Model file for the job. Use its own axes, mm. A direction names the side the tool comes from. Coordinates: 2 decimals unless noted, no trailing zeros. Loops run counter-clockwise (first coordinate to the right, second up) from the corner with the lowest first, then second, coordinate; pieces in that order, holes last. Notation, with made-up numbers: M 83.25,-38 L 110.25,-38 A24 ccw 110.25,-27 Z; hole C 22.25,2.25 d7. An arc over 180 degrees is marked long. One line per question, with ' | ' between items. Start each with the question number.
```python
from build123d import *

# Parameters (mm, degrees)
SKETCH_1_R      = 5
EXTRUDE_1_DEPTH = 3


with BuildPart() as part:
    # 草图1 → 凸台-拉伸1 (new body)
    with BuildSketch(Plane.XY):
        Polygon((-9.837963803, 8.570517693), (60.162036197, 8.570517693), (-9.837963803, -31.429482307), align=None)
        Circle(SKETCH_1_R, mode=Mode.SUBTRACT)
        Polygon((5.831882272, 4.782203257), (5.831882272, -17.086702804), (46.814556623, 4.782203257), align=None, mode=Mode.SUBTRACT)
    extrude(amount=EXTRUDE_1_DEPTH)


solid = part.part
```
(1) Band-saw the part on D-D on y = -11. Write the cut outline in (x, z).
(2) Band-saw the part on C-C on x = 0. Write the cut outline in (y, z), then the cut area to 3 significant figures.
(3) Drill centre lines: line 1 (X direction, y = -2, z = 1.5); line 2 (X direction, y = 2, z = 2); line 3 (X direction, y = -13.5, z = 0.2). Where is each one in solid material? Low to high. Write a range as [from, to].
(4) 3-axis set-ups, long thin cutter, end or side, ignore diameter. For faces 1 (the face through (26.036, -6.305, 1.479)), 2 (the face through (25, 8.571, 1)): which of +Z, -Z, +X, -X, +Y, -Y reach the whole face in a straight line?
(5) Band-saw the part on B-B on y = 0. Write the cut outline in (x, z), then the cut area to 3 significant figures.
(6) Pin check, flat tips, straight feed: P1, Ø0.9, axis at y = -6, z = 1, coming from the +X side; P2, Ø1.5, axis at x = 13, y = 3, coming from the -Z side; P3, Ø1.5, axis at x = 0, y = -8.5, coming from the -Z side; P4, Ø1.5, axis at x = 18.5, z = 2, coming from the -Y side. Stop position of each tip, or through.
(7) Two-plate mould, pull along Z, no slides. Class faces 3 (the face through (5, -5, 3)), 4 (the face through (5, -5, 0)), 5 (the face through (-1.08, -4.88, 1.48)): pulls with the +Z half, pulls with the -Z half, needs draft (parallel to the pull), parting line crosses it, or undercut.
(8) Band-saw the part on A-A on z = 1.6. Write the cut outline in (x, y).
Computed values:
1) outline: M -9.84,0 L 5.83,0 L 5.83,3 L -9.84,3 Z; M 17.24,0 L 25.91,0 L 25.91,3 L 17.24,3 Z
2) outline: M -25.81,0 L -5,0 L -5,3 L -25.81,3 Z; M 5,0 L 8.57,0 L 8.57,3 L 5,3 Z | area: 73.1 mm^2
3) line 1: [-9.84, -4.58], [4.58, 5.83], [34.1, 41.66] | line 2: [-9.84, -4.58], [4.58, 5.83], [41.6, 48.66] | line 3: [-9.84, 5.83], [12.55, 21.54]
4) face 1: +Z, -Z | face 2: +Z, -Z, +X, -X, +Y
5) outline: M -9.84,0 L -5,0 L -5,3 L -9.84,3 Z; M 5,0 L 5.83,0 L 5.83,3 L 5,3 Z; M 37.85,0 L 45.16,0 L 45.16,3 L 37.85,3 Z | area: 38.9 mm^2
6) P1: x = 35.45 | P2: through | P3: z = 0 | P4: y = -15.66
7) face 3: pulls with the +Z half | face 4: pulls with the -Z half | face 5: needs draft
8) outline: M -9.84,-31.43 L 60.16,8.57 L -9.84,8.57 Z; hole C 0,0 d10; hole M 5.83,-17.09 L 46.81,4.78 L 5.83,4.78 Z
